Source: three-view drawing plus pictorial views. Frame: mm from the lowest corner of the part. A direction names the side the tool comes from. Give positions to 0.01 mm unless a question says otherwise; leave off trailing zeros.
1) First-contact query: P1, Ø1, axis at y = 14.5, z = 65, coming from the -X side; P2, Ø7, axis at y = 13, z = 64, coming from the +X side; P3, Ø4, axis at x = 62.69, z = 76.2, coming from the -Y side; P4, Ø13.5, axis at x = 6, z = 32.5, coming from the -Y side. Flat tips, straight axial feed; report the tip coordinate or a pass-through.
2) Section A-A, the plane z = 76.2. Give the number of separate pieces and of enclosed holes in the cut face, plus the area to 3 significant figures.
3) Material intervals for line 1 (X direction, y = 29.9, z = 76.2) (1 decimal); line 2 (X direction, y = 29, z = 25) (1 decimal); line 3 (Y direction, x = 80.5, z = 25.4), sorted ascending.
4) Access query for the marked faces 1, 2 and 3. Directions: +Z, -Z, +X, -X, +Y, -Y. A direction counts if a zero-diameter tool reaches every point of the face in a straight line with its end or side. Return the directions, or none.
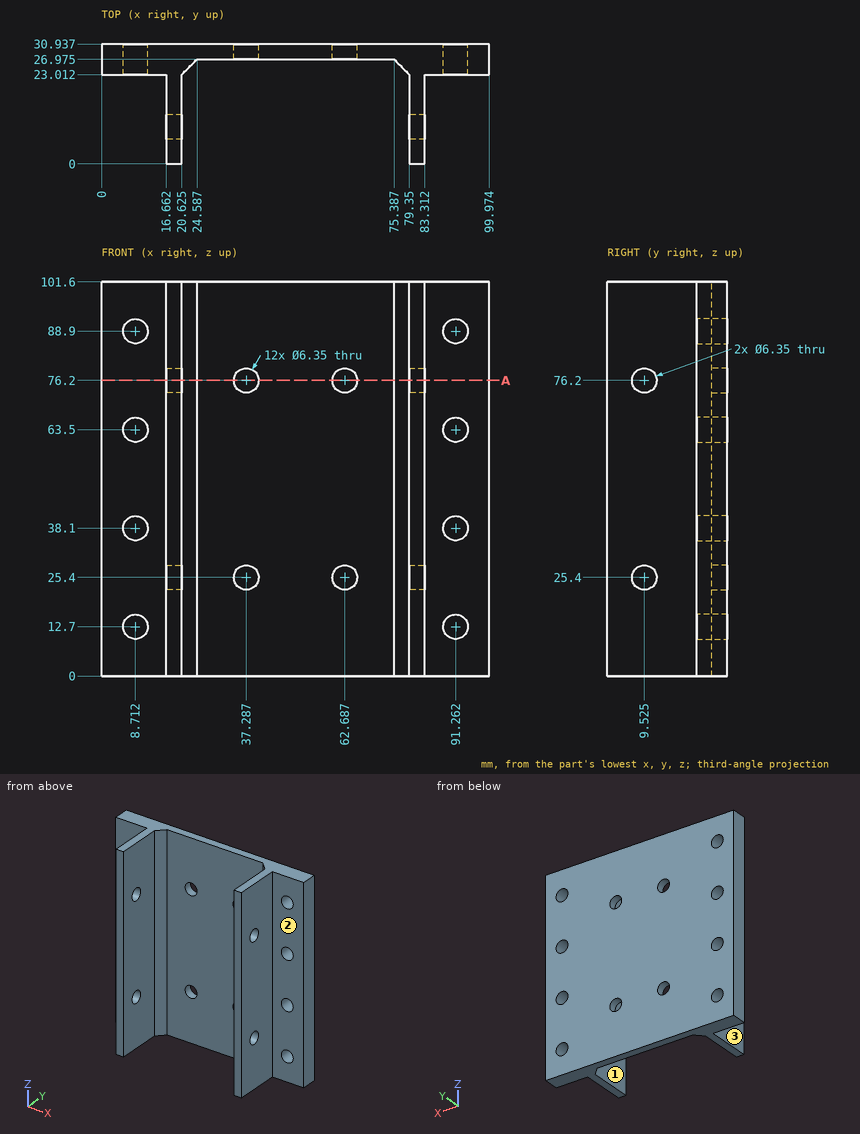
From the geometry:
1. P1: stops at x = 16.66
1. P2: stops at x = 83.31
1. P3: passes through
1. P4: stops at y = 23.01
2. separate pieces: 5
2. enclosed holes: 0
2. area: 657 mm2
3. line 1: x = 0 to 34.1, 40.5 to 59.5, 65.9 to 100
3. line 2: x = 0 to 34.1, 40.4 to 59.5, 65.8 to 100
3. line 3: y = 0 to 6.35, 12.7 to 30.94
4. face 1: +Z, -Z, -Y
4. face 2: +Z, -Z, +X, -Y
4. face 3: +Z, -Z, -X, -Y
